Autodesk Inventor part; units mm, degrees
ref_plane "YZ Plane" through (0, 0, 0) normal (1, 0, 0) x (0, 1, 0)
ref_plane "XZ Plane" through (0, 0, 0) normal (0, 1, 0) x (-1, 0, 0)
ref_plane "XY Plane" through (0, 0, 0) normal (0, 0, 1) x (1, 0, 0)
sketch "スケッチ1" plane through (0, 0, 0) normal (0, 0, 1) x (1, 0, 0)
  line L0 (0, 0) -> (0, -2) construction
  line L1 (-1.6, 0) -> (-1.6, -2)
  line L2 (1.6, -2) -> (1.6, 0)
  arc A0 (1.6, 0) -> (-1.6, 0) centre (0, 0) ccw
  arc A1 (-1.6, -2) -> (1.6, -2) centre (0, -2) ccw
  line L3 (-30, -50) -> (30, -50)
  line L4 (30, -50) -> (30, 50)
  line L5 (30, 50) -> (-30, 50)
  line L6 (-30, 50) -> (-30, -50)
  line L7 (-30, -50) -> (30, 50) construction
  line L8 (30, -50) -> (-30, 50) construction
  line L9 (15, -10) -> (-15, -10) construction
  line L10 (15, -10) -> (15, -12) construction
  line L11 (13.4, -10) -> (13.4, -12)
  line L12 (16.6, -12) -> (16.6, -10)
  arc A2 (16.6, -10) -> (13.4, -10) centre (15, -10) ccw
  arc A3 (13.4, -12) -> (16.6, -12) centre (15, -12) ccw
  line L13 (-15, -10) -> (-15, -12) construction
  line L14 (-16.6, -10) -> (-16.6, -12)
  line L15 (-13.4, -12) -> (-13.4, -10)
  arc A4 (-13.4, -10) -> (-16.6, -10) centre (-15, -10) ccw
  arc A5 (-16.6, -12) -> (-13.4, -12) centre (-15, -12) ccw
  point P0 (0, -1)
  point P1 (15, -11)
  point P2 (-15, -11)
  point P3 (0, -10)
  dimension "d0" = 3.2
  dimension "d1" = 60
  dimension "d2" = 100
  dimension "d5" = 30
  dimension "d6" = 10
  dimension "d7" = 2
extrude "押し出し1" add sketch "スケッチ1" along normal blind 3
sketch "スケッチ2" plane through (0, 0, 3) normal (0, 0, 1) x (1, 0, 0)
  arc A0 (2.0211, 340.4082) -> (8.8067, 38.5424) centre (32.0275, 190.0735) ccw
  circle A1 centre (0, 29.945) radius 10 construction
  circle A2 centre (0, 29.945) radius 5.2
  arc A3 (-13.4, -10) -> (-16.6, -10) centre (-15, -10) ccw
  line L0 (-13.4, -10) -> (-13.4, -12)
  arc A4 (-16.6, -12) -> (-13.4, -12) centre (-15, -12) ccw
  line L1 (-16.6, -12) -> (-16.6, -10)
  arc A5 (16.6, -10) -> (13.4, -10) centre (15, -10) ccw
  line L2 (16.6, -10) -> (16.6, -12)
  arc A6 (13.4, -12) -> (16.6, -12) centre (15, -12) ccw
  line L3 (13.4, -12) -> (13.4, -10)
  arc A7 (1.6, 0) -> (-1.6, 0) centre (0, 0) ccw
  line L4 (1.6, 0) -> (1.6, -2)
  arc A8 (-1.6, -2) -> (1.6, -2) centre (0, -2) ccw
  line L5 (-1.6, -2) -> (-1.6, 0)
  line L6 (-30, -50) -> (30, -50)
  line L7 (30, -50) -> (30, 50)
  line L8 (30, 50) -> (-30, 50)
  line L9 (-30, 50) -> (-30, -50)
  arc A9 (19.6, -10) -> (19.4275, -8.752) centre (15, -10) ccw
  line L10 (19.6, -10) -> (19.6, -12)
  arc A10 (12.2593, -15.6944) -> (19.6, -12) centre (15, -12) ccw
  line L11 (10.4, -12) -> (10.4, -10)
  line L12 (4.6, -2) -> (4.6, 0)
  arc A11 (4.6, 0) -> (-4.6, 0) centre (0, 0) ccw
  line L13 (-4.6, 0) -> (-4.6, -2)
  arc A12 (-4.6, -2) -> (4.6, -2) centre (0, -2) ccw
  arc A13 (-19.4275, -8.752) -> (-19.6, -10) centre (-15, -10) ccw
  line L14 (-10.4, -10) -> (-10.4, -12)
  arc A14 (-19.6, -12) -> (-12.2593, -15.6944) centre (-15, -12) ccw
  line L15 (-19.6, -12) -> (-19.6, -10)
  arc A15 (7.8924, 32.1697) -> (-7.8924, 32.1697) centre (0, 29.945) ccw
  line L16 (19.4275, -8.752) -> (7.8924, 32.1697)
  line L17 (-19.4275, -8.752) -> (-7.8924, 32.1697)
  line L18 (0, -6.6) -> (12.2593, -15.6944)
  line L19 (0, -6.6) -> (-12.2593, -15.6944)
  dimension "d8" = 20
  dimension "d9" = 10.4
  dimension "d10" = 3
  dimension "d11" = 3
  dimension "d12" = 3
  dimension "d13" = 3
extrude "押し出し2" cut sketch "スケッチ2" against normal blind 3 contours A12 L13 A11 L12 | L10 A10 L18 L19 A14 L15 A13 L17 A15 L16 A9 keep common part
fillet "フィレット1" radius 2 1 edges at (0, -6.6, 1.5)
properties part number "POT2BASE"
The model under review builds one solid part; all positions refer to its coordinate system, in mm. A direction names the side the tool comes from. Round coordinates to 2 decimals unless told otherwise and drop trailing zeros. Order: outer loops, then holes, each group sorted by start corner. A loop starts at its lowest first (then second) coordinate and runs counter-clockwise, first axis right, second up.
Item 1: For pin 1 (1.5 mm diameter, centred on y = 24, z = 2, fed in from +X); pin 2 (1 mm diameter, centred on y = -1, z = 1.5, fed in from -X), all flat-tipped, find the tip position at first contact; note any pin that passes through.
Working result:
pin 1: stops at x = 10.41
pin 2: stops at x = -17.38
Item 2: Add section D-D, the plane z = 0.9. State the section outline as (x, y) points (1 decimal).
Working result:
outline: (-19.6, -12) arc R4.6 ccw to (-12.3, -15.7) - (-1.2, -7.5) arc R2 cw to (1.2, -7.5) - (12.3, -15.7) arc R4.6 ccw to (19.6, -12) - (19.6, -10) arc R4.6 ccw to (19.4, -8.8) - (7.9, 32.2) arc R8.2 ccw to (-7.9, 32.2) - (-19.4, -8.8) arc R4.6 ccw to (-19.6, -10) - close; hole (-16.6, -12) arc R1.6 ccw to (-13.4, -12) - (-13.4, -10) arc R1.6 ccw to (-16.6, -10) - close; hole circle Ø10.4 at (0, 29.9); hole (-1.6, -2) arc R1.6 ccw to (1.6, -2) - (1.6, 0) arc R1.6 ccw to (-1.6, 0) - close; hole (13.4, -12) arc R1.6 ccw to (16.6, -12) - (16.6, -10) arc R1.6 ccw to (13.4, -10) - close
Item 3: Draft analysis for pull direction Y (two halves, no side actions). For faces 4 (the cylindrical face through (17.004, -16.14, 1.521)), 5 (the cylindrical face through (0.149, 38.144, 1.521)), 6 (the cylindrical face through (15, -8.4, 1.5)), state which applies: released by +Y, released by -Y, zero draft, split by the parting line, or undercut.
Working result:
face 4: released by -Y
face 5: released by +Y
face 6: undercut
Item 4: To check wall thickness, follow probe 1 along Y at (x, z) = (0, 2.2) (3 decimals); probe 2 along X at (y, z) = (-12.5, 2.1); probe 3 along X at (y, z) = (26.5, 2.2). State the ranges of each line that lie inside material, in increasing order.
Working result:
probe 1: y = -7.09 to -3.6, 1.6 to 24.745, 35.145 to 38.145
probe 2: x = -19.57 to -16.52, -13.48 to -7.95, 7.95 to 13.48, 16.52 to 19.57
probe 3: x = -9.49 to -3.9, 3.9 to 9.49
Item 5: Add section B-B, the plane y = 31.5. State the section outline as (x, z) points.
Working result:
outline: (-8.08, 0) - (-4.96, 0) - (-4.96, 3) - (-8.08, 3) - close; (4.96, 0) - (8.08, 0) - (8.08, 3) - (4.96, 3) - close
Item 6: Add section C-C, the plane x = -15. State the section outline as (y, z) points.
Working result:
outline: (-16.6, 0) - (-13.6, 0) - (-13.6, 3) - (-16.6, 3) - close; (-8.4, 0) - (6.95, 0) - (6.95, 3) - (-8.4, 3) - close
Item 7: Add section A-A, the plane x = 0. State the section outline as (y, z) points (3 decimals).
Working result:
outline: (-7.09, 0) - (-3.6, 0) - (-3.6, 3) - (-7.09, 3) - close; (1.6, 0) - (24.745, 0) - (24.745, 3) - (1.6, 3) - close; (35.145, 0) - (38.145, 0) - (38.145, 3) - (35.145, 3) - close
Item 8: Machinability: for faces 1 (the flat face through (0, 5, 0)), 2 (the cylindrical face through (0, 1.6, 1.5)), 3 (the flat face through (6.648, -11.532, 1.521)), which of the approach directions +Z, -Z, +X, -X, +Y, -Y give a long, thin tool a straight path to every point of the face, cutting with its end or side? Answer none if there is none.
Working result:
face 1: -Z, +X, -X, +Y, -Y
face 2: +Z, -Z
face 3: +Z, -Z, -Y
